Could you check a few things on this model? Use its own coordinates, in mm. A direction names the side the tool comes from. Give positions to 0.01 mm unless a question says otherwise; leave off trailing zeros. Order: outer loops, then holes, each group sorted by start corner. A loop starts at its lowest first (then second) coordinate and runs counter-clockwise, first axis right, second up. Notation, with made-up numbers: (-37, -37.5) -> (11, -37.5) arc R8 cw to (11, -32.5) -> close; hole circle Ø4 at (55, 17.25). An arc over 180 degrees is marked (long way). Answer as CSV lines item,"result". Start each with the question number.
(1) I want a section at D-D (x = 15.5). Please give me the cut outline in (y, z).
(2) I want a section at A-A (z = 7.5). Please give me the cut outline in (x, y).
(3) I need wall thicknesses on L1, parallel to X at y = -14, z = 2; L2, parallel to X at y = -18.75, z = 16; L3, parallel to Y at x = 18.5, z = 5. Which ranges of each line are inside material? Lowest first, please.
(4) On a 3-axis mill with a long thin cutter (end or side, diameter ignored), from which of +Z, -Z, +X, -X, +Y, -Y can I reach the whole of each face in a straight line? I mean faces 1 (the face through (10, -6.35, 3)), 2 (the face through (9, -16, 12.7)), 3 (the face through (9, -22, 19.05)), 4 (the face through (3, -16, 19.05)). Say none if no direction works.
(5) I want a section at B-B (y = -21.25). Please give me the cut outline in (x, z), plus the area to 3 significant figures.
(6) I want a section at C-C (x = 5.25). Please give me the cut outline in (y, z), plus the area to 3 significant figures.
(7) Will these pins go through, and if not, where does the flat tip stop? pin 1 Ø1.9 at (y, z) = (-15, 10) entering from +X; pin 2 Ø1.9 at (x, y) = (16, -23) entering from +Z; pin 3 Ø7 at (x, z) = (10, 8.5) entering from +Y.
```python
from build123d import *

# Parameters (mm, degrees)
F1_DEPTH = 6.35
F3_DEPTH = 6.35
F5_DEPTH = 6.35
F6_W     = 6.35
F6_H     = 6.35
F7_DEPTH = 6.35


with BuildPart() as f1:
    # F0 (on Top) → F1 (new body)
    with BuildSketch(Plane.XY):
        Polygon((0, 0), (0, -25.4), (25.4, -25.4), (25.4, -19.05), (19.05, -19.05), (19.05, -12.7), (12.7, -12.7), (12.7, -6.35), (6.35, -6.35), (6.35, 0), align=None)
    extrude(amount=F1_DEPTH)

    # F2 (on face) → F3 (join)
    with BuildSketch(Plane.XY.offset(6.35)):
        Polygon((6.35, -6.35), (0, -6.35), (0, -25.4), (19.05, -25.4), (19.05, -19.05), (12.7, -19.05), (12.7, -12.7), (6.35, -12.7), align=None)
    extrude(amount=F3_DEPTH)

    # F4 (on face) → F5 (join)
    with BuildSketch(Plane.XY.offset(12.7)):
        Polygon((6.35, -12.7), (0, -12.7), (0, -25.4), (12.7, -25.4), (12.7, -19.05), (6.35, -19.05), align=None)
    extrude(amount=F5_DEPTH)

    # F6 (on face) → F7 (join)
    with BuildSketch(Plane.XY.offset(19.05)):
        with Locations((3.175, -22.225)):
            Rectangle(F6_W, F6_H)
    extrude(amount=F7_DEPTH)


solid = f1.part
```
Final values:
1,outline,"(-25.4, 0) -> (-12.7, 0) -> (-12.7, 6.35) -> (-19.05, 6.35) -> (-19.05, 12.7) -> (-25.4, 12.7) -> close"
2,outline,"(0, -25.4) -> (19.05, -25.4) -> (19.05, -19.05) -> (12.7, -19.05) -> (12.7, -12.7) -> (6.35, -12.7) -> (6.35, -6.35) -> (0, -6.35) -> close"
3,L1,"0 to 19.05"
3,L2,"0 to 6.35"
3,L3,"-25.4 to -12.7"
4,face 1,"+Z, -Z, +X, +Y"
4,face 2,"+Z, +X, +Y"
4,face 3,"+Z, +X, +Y, -Y"
4,face 4,"+Z, +X, -X, +Y"
5,outline,"(0, 0) -> (25.4, 0) -> (25.4, 6.35) -> (19.05, 6.35) -> (19.05, 12.7) -> (12.7, 12.7) -> (12.7, 19.05) -> (6.35, 19.05) -> (6.35, 25.4) -> (0, 25.4) -> close"
5,area,"403 mm²"
6,outline,"(-25.4, 0) -> (0, 0) -> (0, 6.35) -> (-6.35, 6.35) -> (-6.35, 12.7) -> (-12.7, 12.7) -> (-12.7, 19.05) -> (-19.05, 19.05) -> (-19.05, 25.4) -> (-25.4, 25.4) -> close"
6,area,"403 mm²"
7,pin 1,"x = 12.7"
7,pin 2,"z = 12.7"
7,pin 3,"y = -6.35"
